Source: CAD feature listing. Evaluate the final solid. Frame: model axes, mm. Coordinates: 2 decimals unless noted, no trailing zeros. Write each loop counter-clockwise with the first axis right and the second up, starting at its lowest first coordinate (ties: lowest second). Pieces come first, ordered by that corner, then holes. Notation, with made-up numbers: M 13,-36.75 L 48,-36.75 A30 cw 48,-6.75 Z; hole C 67.25,4 d11. An arc over 180 degrees is marked long. One line per item, written item: value. Start each with the question number.
Item 1: Cut plane B-B, the plane z = 58. Output: boundary loops of the cut face in (x, y), then the cut area to 4 significant figures.
Item 2: Pin query (flat end, axial travel): P1, Ø5.5, axis at x = 213.24, z = 253.71, coming from the -Y side; P2, Ø4, axis at x = 72.5, z = 184, coming from the -Y side. Return the tip coordinate at first contact, or that it passes through.
Item 3: Ray query, L1, parallel to Z at x = 222, y = 0.05; L2, parallel to X at y = 0.5, z = 253; L3, parallel to X at y = 0.55, z = 208. Return the intervals inside material, ascending. Write a range as from..to.
Item 4: Mould query, pull axis Y, two halves, no side actions, for faces 1 (the flat face through (91, 1, 132)), 2 (the flat face through (91, 0, 132)). Classes: released by +Y, released by -Y, zero draft, split by the parting line, or undercut.
Item 5: Cut plane A-A, the plane y = 0.65. Output: boundary loops of the cut face in (x, z).
```python
from build123d import *

# Parameters (mm, degrees)
SKETCH_1_W          = 300
SKETCH_1_H          = 300
EXTRUDE_1_DEPTH     = 1
SKETCH_2_R          = 3
CUT_EXTRUDE_2_DEPTH = 374.714004721
SKETCH_3_W          = 44.5
SKETCH_3_H          = 42
CUT_EXTRUDE_4_DEPTH = 374.714004721


with BuildPart() as part:
    # 草图1 → 凸台-拉伸1 (new body)
    with BuildSketch(Plane(origin=(0, 0, 0), x_dir=(1, 0, 0), z_dir=(0, 1, 0))):
        with Locations((93.243141409, -133.714524624)):
            Rectangle(SKETCH_1_W, SKETCH_1_H)
    extrude(amount=EXTRUDE_1_DEPTH)

    # 草图2 → 切除-拉伸2 (cut, through all)
    with BuildSketch(Plane(origin=(0, 0, 0), x_dir=(1, 0, 0), z_dir=(0, 1, 0))):
        with Locations(Location((-26.756858591, -13.714524624, 0), (0, 0, 270))):
            Circle(SKETCH_2_R)
        with Locations(Location((213.243141409, -13.714524624, 0), (0, 0, 270))):
            Circle(SKETCH_2_R)
        with Locations(Location((213.243141409, -253.714524624, 0), (0, 0, 270))):
            Circle(SKETCH_2_R)
        with Locations(Location((-26.756858591, -253.714524624, 0), (0, 0, 270))):
            Circle(SKETCH_2_R)
    extrude(amount=CUT_EXTRUDE_2_DEPTH, mode=Mode.SUBTRACT)

    # 草图3 → 切除-拉伸4 (cut, through all)
    with BuildSketch(Plane(origin=(0, 0, 0), x_dir=(1, 0, 0), z_dir=(0, 1, 0))):
        with Locations((220.993141409, -208.214524624)):
            Rectangle(SKETCH_3_W, SKETCH_3_H)
        with Locations((220.993141409, -59.214524624)):
            Rectangle(SKETCH_3_W, SKETCH_3_H)
    extrude(amount=CUT_EXTRUDE_4_DEPTH, mode=Mode.SUBTRACT)


solid = part.part
```
From the geometry:
1. outline: M -56.76,0 L 198.74,0 L 198.74,1 L -56.76,1 Z
1. area: 255.5 mm²
2. P1: passes through
2. P2: stops at y = 0
3. L1: z = -16.29..38.21, 80.21..187.21, 229.21..283.71
3. L2: x = -56.76..-29.67, -23.84..210.33, 216.16..243.24
3. L3: x = -56.76..198.74
4. face 1: released by +Y
4. face 2: released by -Y
5. outline: M -56.76,-16.29 L 243.24,-16.29 L 243.24,38.21 L 198.74,38.21 L 198.74,80.21 L 243.24,80.21 L 243.24,187.21 L 198.74,187.21 L 198.74,229.21 L 243.24,229.21 L 243.24,283.71 L -56.76,283.71 Z; hole C -26.76,13.71 d6; hole C -26.76,253.71 d6; hole C 213.24,13.71 d6; hole C 213.24,253.71 d6
